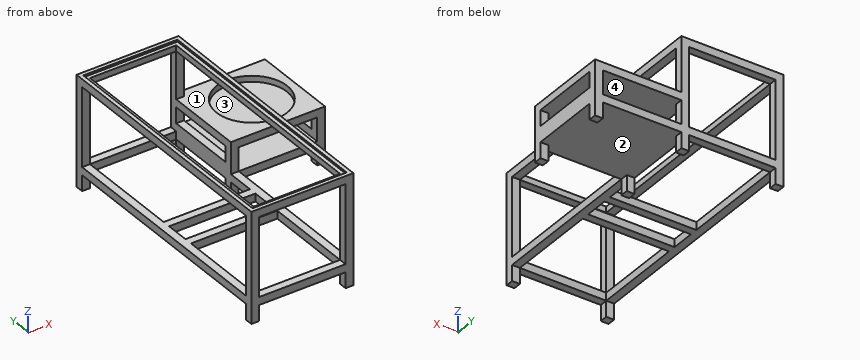
```python
from build123d import *

# Parameters (mm, degrees)
F0_W       = 1320.8
F0_H       = 1625.6
F0_W_2     = 1219.2
F0_H_2     = 1524
F1_DEPTH   = 50.8
F2_W       = 50.8
F2_H       = 50.8
F3_DEPTH   = 508
F4_W       = 1320.8
F4_H       = 1625.6
F4_W_2     = 1219.2
F4_H_2     = 1524
F5_DEPTH   = 50.8
F6_W       = 609.6
F6_H       = 50.8
F7_DEPTH   = 1524
F9_DEPTH   = 609.601
F10_W      = 50.8
F10_H      = 50.8
F11_DEPTH  = 508
F12_W      = 50.8
F12_H      = 50.8
F13_DEPTH  = 1524
F14_W      = 558.8
F14_H      = 254
F15_DEPTH  = 558.8
F15_FACE_W = 508
F15_FACE_H = 203.2
F16_DEPTH  = 50.8
F17_W      = 508.634997
F17_H      = 152.4
F18_DEPTH  = 558.801
F19_W      = 457.139586
F19_H      = 101.6
F20_DEPTH  = 609.601
F21_W      = 609.6
F21_H      = 1574.8
F22_DEPTH  = 12.7
F23_W      = 558.8
F23_H      = 1524
F24_DEPTH  = 596.901
F25_W      = 50.8
F25_H      = 50.8
F26_DEPTH  = 101.6
F27_W      = 50.8
F27_H      = 50.8
F28_DEPTH  = 558.8
F29_R      = 228.6
F30_DEPTH  = 38.1


with BuildPart() as f1:
    # F0 (on Top) → F1 (new body)
    with BuildSketch(Plane.XY):
        Rectangle(F0_W, F0_H)
        Rectangle(F0_W_2, F0_H_2, mode=Mode.SUBTRACT)
    extrude(amount=F1_DEPTH)

    # F2 (on face) → F3 (join)
    with BuildSketch(Plane.XY.offset(50.8)):
        with Locations((-635, 787.4)):
            Rectangle(F2_W, F2_H)
        with Locations((635, 787.4)):
            Rectangle(F2_W, F2_H)
        with Locations((635, -787.4)):
            Rectangle(F2_W, F2_H)
        with Locations((-635, -787.4)):
            Rectangle(F2_W, F2_H)
    extrude(amount=F3_DEPTH)

    # F4 (on face) → F5 (join)
    with BuildSketch(Plane.XY.offset(558.8)):
        Rectangle(F4_W, F4_H)
        Rectangle(F4_W_2, F4_H_2, mode=Mode.SUBTRACT)
    extrude(amount=F5_DEPTH)

    # F6 (on face) → F7 (join, through all)
    with BuildSketch(Plane.XZ.offset(-762)):
        with Locations((-304.8, 584.2)):
            Rectangle(F6_W, F6_H)
    extrude(amount=F7_DEPTH)

    # F8 (on face) → F9 (cut, through all)
    with BuildSketch(Plane.XY.offset(609.6)):
        Polygon((0, 812.8), (0, 762), (0, -812.8), (660.4, -812.8), (660.4, 812.8), align=None)
    extrude(amount=-F9_DEPTH, mode=Mode.SUBTRACT)

    # F10 (on face) → F11 (join, through all)
    with BuildSketch(Plane.XY.offset(50.8)):
        with Locations((-25.4, 787.4)):
            Rectangle(F10_W, F10_H)
        with Locations((-25.4, -787.4)):
            Rectangle(F10_W, F10_H)
    extrude(amount=F11_DEPTH)

    # F12 (on face) → F13 (join, through all)
    with BuildSketch(Plane.XZ.offset(-762)):
        with Locations((-25.4, 25.4)):
            Rectangle(F12_W, F12_H)
    extrude(amount=F13_DEPTH)

    # F14 (on face) → F15 (join)
    with BuildSketch(Plane.YZ):
        with Locations((533.4, 127)):
            Rectangle(F14_W, F14_H)
    extrude(amount=F15_DEPTH)

    # F15_face (on face) → F16 (join)
    with BuildSketch(Plane(origin=(0, 508, 152.4), x_dir=(0, 1, 0), z_dir=(-1, 0, 0))):
        Rectangle(F15_FACE_W, F15_FACE_H)
    extrude(amount=F16_DEPTH)

    # F17 (on face) → F18 (cut, through all)
    with BuildSketch(Plane.XZ.offset(-254)):
        with Locations((253.682502, 127)):
            Rectangle(F17_W, F17_H)
    extrude(amount=-F18_DEPTH, mode=Mode.SUBTRACT)

    # F19 (on face) → F20 (cut, through all)
    with BuildSketch(Plane(origin=(-50.8, 0, 0), x_dir=(0, -1, 0), z_dir=(-1, 0, 0))):
        with Locations((-533.369793, 152.4)):
            Rectangle(F19_W, F19_H)
    extrude(amount=-F20_DEPTH, mode=Mode.SUBTRACT)

    # F21 (on face) → F22 (cut)
    with BuildSketch(Plane.XY.offset(609.6)):
        with Locations((-330.2, 0)):
            Rectangle(F21_W, F21_H)
    extrude(amount=-F22_DEPTH, mode=Mode.SUBTRACT)

    # F23 (on face) → F24 (cut, through all)
    with BuildSketch(Plane.XY.offset(596.9)):
        with Locations((-330.2, 0)):
            Rectangle(F23_W, F23_H)
    extrude(amount=-F24_DEPTH, mode=Mode.SUBTRACT)

    # F25 (on face) → F26 (join)
    with BuildSketch(Plane(origin=(0, 0, 0), x_dir=(1, 0, 0), z_dir=(0, 0, -1))):
        with Locations((-635, 787.4)):
            Rectangle(F25_W, F25_H)
        with Locations((-25.4, 787.4)):
            Rectangle(F25_W, F25_H)
        with Locations((-635, -787.4)):
            Rectangle(F25_W, F25_H)
        with Locations((-25.4, -787.4)):
            Rectangle(F25_W, F25_H)
        with Locations((-25.4, -279.4)):
            Rectangle(F25_W, F25_H)
        with Locations((533.4, -279.4)):
            Rectangle(F25_W, F25_H)
        with Locations((533.4, -787.4)):
            Rectangle(F25_W, F25_H)
    extrude(amount=F26_DEPTH)

    # F27 (on face) → F28 (join, through all)
    with BuildSketch(Plane.YZ.offset(-609.6)):
        with Locations((-152.4, 25.4)):
            Rectangle(F27_W, F27_H)
        with Locations((50.8, 25.4)):
            Rectangle(F27_W, F27_H)
    extrude(amount=F28_DEPTH)

    # F29 (on face) → F30 (cut)
    with BuildSketch(Plane.XY.offset(254)):
        with Locations((279.4, 533.4)):
            Circle(F29_R)
    extrude(amount=-F30_DEPTH, mode=Mode.SUBTRACT)


solid = f1.part
```
Geometry check sheet. Reference: the model listing, model coordinates, mm. Face numbers are marked on the shaded views. A direction names the side the tool comes from. Coordinates: 2 decimals unless noted, no trailing zeros. Loops run counter-clockwise (first coordinate to the right, second up) from the corner with the lowest first, then second, coordinate; pieces in that order, holes last. Notation, with made-up numbers: (-19.75, 53.5) -> (29.25, 53.5) arc R20 cw to (29.25, 79.5) -> close; hole circle Ø3 at (45.25, 12). An arc over 180 degrees is marked (long way). Put each result on its own line as item: value.
1) Cross-section at B-B on x = 279.4. Record the boundary of the cut face in (y, z).
Result set:
outline: (254, 0) -> (812.8, 0) -> (812.8, 50.8) -> (254, 50.8) -> close; (254, 203.2) -> (812.8, 203.2) -> (812.8, 254) -> (762, 254) -> (762, 215.9) -> (304.8, 215.9) -> (304.8, 254) -> (254, 254) -> close
2) Cross-section at D-D on x = -117.5. Record the boundary of the cut face in (y, z), plus the area to 3 significant figures.
Result set:
outline: (-812.8, 0) -> (-762, 0) -> (-762, 50.8) -> (-812.8, 50.8) -> close; (-812.8, 558.8) -> (-762, 558.8) -> (-762, 596.9) -> (-787.4, 596.9) -> (-787.4, 609.6) -> (-812.8, 609.6) -> close; (-177.8, 0) -> (-127, 0) -> (-127, 50.8) -> (-177.8, 50.8) -> close; (25.4, 0) -> (76.2, 0) -> (76.2, 50.8) -> (25.4, 50.8) -> close; (762, 0) -> (812.8, 0) -> (812.8, 50.8) -> (762, 50.8) -> close; (762, 558.8) -> (812.8, 558.8) -> (812.8, 609.6) -> (787.4, 609.6) -> (787.4, 596.9) -> (762, 596.9) -> close
area: 14,800 mm^2
3) Release check for a two-part mould opening along X. For the marked faces 1 and 2 record: released by +X, released by -X, zero draft, split by the parting line, or undercut.
Result set:
face 1: zero draft
face 2: undercut
4) Gauge pin test, flat end, axial feed: pin 1 Ø8 at (x, y) = (151.5, 525.5) entering from -Z. Record the tip position at first contact, or that the pin passes through.
Result set:
pin 1: stops at z = 0
5) Cross-section at A-A on y = -345. Record the boundary of the cut face in (x, z).
Result set:
outline: (-660.4, 0) -> (-609.6, 0) -> (-609.6, 50.8) -> (-660.4, 50.8) -> close; (-660.4, 558.8) -> (-609.6, 558.8) -> (-609.6, 596.9) -> (-635, 596.9) -> (-635, 609.6) -> (-660.4, 609.6) -> close; (-50.8, 0) -> (0, 0) -> (0, 50.8) -> (-50.8, 50.8) -> close; (-50.8, 558.8) -> (0, 558.8) -> (0, 609.6) -> (-25.4, 609.6) -> (-25.4, 596.9) -> (-50.8, 596.9) -> close
6) Cross-section at C-C on z = 398.5. Record the boundary of the cut face in (x, y), plus the area to 3 significant figures.
Result set:
outline: (-660.4, -812.8) -> (-609.6, -812.8) -> (-609.6, -762) -> (-660.4, -762) -> close; (-660.4, 762) -> (-609.6, 762) -> (-609.6, 812.8) -> (-660.4, 812.8) -> close; (-50.8, -812.8) -> (0, -812.8) -> (0, -762) -> (-50.8, -762) -> close; (-50.8, 762) -> (0, 762) -> (0, 812.8) -> (-50.8, 812.8) -> close
area: 10,300 mm^2
7) Tool access check on the marked faces 3 and 4. Record the directions out of +Z, -Z, +X, -X, +Y, -Y that give a thin tool (end or side, any length) a straight path to the whole face; none if there is none.
Result set:
face 3: +Z
face 4: none
8) Thickness scan on line 1 (Y direction, x = 279.4, z = 227.5); line 2 (X direction, y = -212, z = 26); line 3 (Z direction, x = 296, y = 612.5). Record the ranges inside material, lowest first.
Result set:
line 1: y = 254 to 304.8, 762 to 812.8
line 2: x = -660.4 to -609.6, -50.8 to 0
line 3: z = 0 to 50.8, 203.2 to 215.9
